Geometry check sheet. Reference: the model listing, model coordinates, mm. A direction names the side the tool comes from. Give positions to 0.01 mm unless a question says otherwise; leave off trailing zeros. Write each loop counter-clockwise with the first axis right and the second up, starting at its lowest first coordinate (ties: lowest second). Pieces come first, ordered by that corner, then holes.
(1) Cross-section at A-A (y = 5.2). Record the boundary of the cut face in (x, z), and give its area (3 significant figures).
(2) Depth check by flat-ended pin: P1, Ø3, axis at y = 6.5, z = 6, coming from the +X side; P2, Ø3.5, axis at x = 9, z = 5, coming from the +Y side; P3, Ø4, axis at x = 58, y = 7, coming from the +Z side. Enter the tip coordinate at first touch or a pass-through.
(3) Mould release check, pull along X, two halves, no side actions. Record for faces 1 (the flat face through (28, 1, 0.9)), 2 (the flat face through (0, 4, 4)), 3 (the flat face through (36, 0, 4)): +X half, -X half, draft (parallel to the pull), parting line (faces both ways), or undercut.
(4) Cross-section at C-C (z = 1.5). Record the boundary of the cut face in (x, y).
(5) Cross-section at B-B (x = 51). Record the boundary of the cut face in (y, z).
(6) Tool access check on faces 4 (the flat face through (64, 3, 5.3)), 5 (the flat face through (17.5, 3, 4)), 6 (the cylindrical face through (69.8, 1, 3.8)). Record the directions out of +Z, -Z, +X, -X, +Y, -Y that give a thin tool (end or side, any length) a straight path to the whole face; none if there is none.
(7) Thickness scan on line 1 along X through (y, z) = (4.5, 1); line 2 along Y through (x, z) = (2.2, 5.7); line 3 along X through (y, z) = (1.5, 1.25). Record the ranges inside material, lowest first.
```python
from build123d import *

# Parameters (mm, degrees)
BOSS_EXTRUDE1_DEPTH = 7.4
CUT_EXTRUDE1_DEPTH  = 10
CUT_EXTRUDE2_DEPTH  = 2
CUT_EXTRUDE3_REACH  = 72.8
SKETCH5_R           = 0.75
CUT_EXTRUDE4_DEPTH  = 10
CUT_EXTRUDE6_DEPTH  = 0.7


with BuildPart() as part:
    # Sketch1 → Boss-Extrude1 (new body)
    with BuildSketch(Plane.XY):
        Polygon((0, 0), (0, 8.8), (3, 8.8), (3, 2), (17.5, 2), (17.5, 3.85), (40, 3.85), (40, 8.8), (43, 8.8), (43, 2), (57.5, 2), (57.5, 3.85), (70.8, 3.85), (70.8, 0), align=None)
    extrude(amount=BOSS_EXTRUDE1_DEPTH)

    # Sketch3 → Cut-Extrude1 (cut)
    with BuildSketch(Plane(origin=(0, 3.85, 0), x_dir=(1, 0, 0), z_dir=(0, 1, 0))):
        with BuildLine():
            Line((30.5, -5.3), (24.5, -5.3))
            ThreePointArc((24.5, -5.3), (22.9, -3.7), (24.5, -2.1))
            Line((24.5, -2.1), (30.5, -2.1))
            ThreePointArc((30.5, -2.1), (32.1, -3.7), (30.5, -5.3))
        make_face()
        with BuildLine():
            Line((67, -5.3), (61, -5.3))
            ThreePointArc((61, -5.3), (59.4, -3.7), (61, -2.1))
            Line((61, -2.1), (67, -2.1))
            ThreePointArc((67, -2.1), (68.6, -3.7), (67, -5.3))
        make_face()
    extrude(amount=-CUT_EXTRUDE1_DEPTH, mode=Mode.SUBTRACT)

    # Sketch4 → Cut-Extrude2 (cut)
    with BuildSketch(Plane.XZ):
        with BuildLine():
            Line((24.5, 6.5), (30.5, 6.5))
            ThreePointArc((30.5, 6.5), (33.3, 3.7), (30.5, 0.9))
            Line((30.5, 0.9), (24.5, 0.9))
            ThreePointArc((24.5, 0.9), (21.7, 3.7), (24.5, 6.5))
        make_face()
        with BuildLine():
            Line((24.5, 5.3), (30.5, 5.3))
            ThreePointArc((30.5, 5.3), (32.1, 3.7), (30.5, 2.1))
            Line((30.5, 2.1), (24.5, 2.1))
            ThreePointArc((24.5, 2.1), (22.9, 3.7), (24.5, 5.3))
        make_face(mode=Mode.SUBTRACT)
        with BuildLine():
            Line((61, 6.5), (67, 6.5))
            ThreePointArc((67, 6.5), (69.8, 3.7), (67, 0.9))
            Line((67, 0.9), (61, 0.9))
            ThreePointArc((61, 0.9), (58.2, 3.7), (61, 6.5))
        make_face()
        with BuildLine():
            Line((61, 5.3), (67, 5.3))
            ThreePointArc((67, 5.3), (68.6, 3.7), (67, 2.1))
            Line((67, 2.1), (61, 2.1))
            ThreePointArc((61, 2.1), (59.4, 3.7), (61, 5.3))
        make_face(mode=Mode.SUBTRACT)
    extrude(amount=-CUT_EXTRUDE2_DEPTH, mode=Mode.SUBTRACT)

    # Sketch5 → Cut-Extrude3 (cut, up to next)
    with BuildSketch(Plane.ZY, mode=Mode.PRIVATE) as cut_extrude3_sk1:
        with Locations((5.7, 5.2)):
            Circle(SKETCH5_R)
    cut_extrude3_tool1 = extrude(cut_extrude3_sk1.sketch, amount=-CUT_EXTRUDE3_REACH, mode=Mode.PRIVATE) & part.part
    add(cut_extrude3_tool1.solids().sort_by_distance((0, 5.2, 5.7))[0], mode=Mode.SUBTRACT)

    # Sketch6 → Cut-Extrude4 (cut)
    with BuildSketch(Plane.XZ):
        with BuildLine():
            Line((67.1, 0), (70.8, 0))
            Line((70.8, 0), (70.8, 3.7))
            ThreePointArc((70.8, 3.7), (69.71629509, 1.08370491), (67.1, 0))
        make_face()
        with BuildLine():
            ThreePointArc((67.1, 7.4), (69.71629509, 6.31629509), (70.8, 3.7))
            Line((70.8, 3.7), (70.8, 7.4))
            Line((70.8, 7.4), (67.1, 7.4))
        make_face()
    extrude(amount=-CUT_EXTRUDE4_DEPTH, mode=Mode.SUBTRACT)

    # Sketch8 → Cut-Extrude6 (cut)
    with BuildSketch(Plane(origin=(0, 2, 0), x_dir=(1, 0, 0), z_dir=(0, 1, 0))):
        with BuildLine():
            Line((7.8, -2.75), (14.8, -2.75))
            ThreePointArc((14.8, -2.75), (16.3, -4.25), (14.8, -5.75))
            Line((14.8, -5.75), (7.8, -5.75))
            ThreePointArc((7.8, -5.75), (6.3, -4.25), (7.8, -2.75))
        make_face()
        with BuildLine():
            Line((47.8, -2.75), (54.8, -2.75))
            ThreePointArc((54.8, -2.75), (56.3, -4.25), (54.8, -5.75))
            Line((54.8, -5.75), (47.8, -5.75))
            ThreePointArc((47.8, -5.75), (46.3, -4.25), (47.8, -2.75))
        make_face()
    extrude(amount=-CUT_EXTRUDE6_DEPTH, mode=Mode.SUBTRACT)


solid = part.part
```
Reply:
1. outline: (0, 0) - (3, 0) - (3, 4.95) - (0, 4.95) - close; (0, 6.45) - (3, 6.45) - (3, 7.4) - (0, 7.4) - close; (40, 0) - (43, 0) - (43, 7.4) - (40, 7.4) - close
1. area: 39.9 mm2
2. P1: stops at x = 43
2. P2: stops at y = 2
2. P3: passes through
3. face 1: undercut
3. face 2: -X half
3. face 3: draft
4. outline: (0, 0) - (22.77, 0) - (22.77, 2) - (32.23, 2) - (32.23, 0) - (59.27, 0) - (59.27, 2) - (68.73, 2) - (68.73, 0) - (70.07, 0) - (70.07, 3.85) - (57.5, 3.85) - (57.5, 2) - (43, 2) - (43, 8.8) - (40, 8.8) - (40, 3.85) - (17.5, 3.85) - (17.5, 2) - (3, 2) - (3, 8.8) - (0, 8.8) - close
5. outline: (0, 0) - (2, 0) - (2, 2.75) - (1.3, 2.75) - (1.3, 5.75) - (2, 5.75) - (2, 7.4) - (0, 7.4) - close
6. face 4: +Y, -Y
6. face 5: +Z, -Z, +Y
6. face 6: -Y
7. line 1: x = 0 to 3, 40 to 43
7. line 2: y = 0 to 4.45, 5.95 to 8.8
7. line 3: x = 0 to 23.14, 31.86 to 59.64, 68.36 to 69.87
